The listing builds one solid part. Answer for the finished solid, in the listing's coordinates (mm). Face numbers are marked on the shaded views. A direction names the side the tool comes from. Coordinates: 2 decimals unless noted, no trailing zeros. Write each loop counter-clockwise with the first axis right and the second up, starting at its lowest first coordinate (ties: lowest second). Pieces come first, ordered by that corner, then holes.
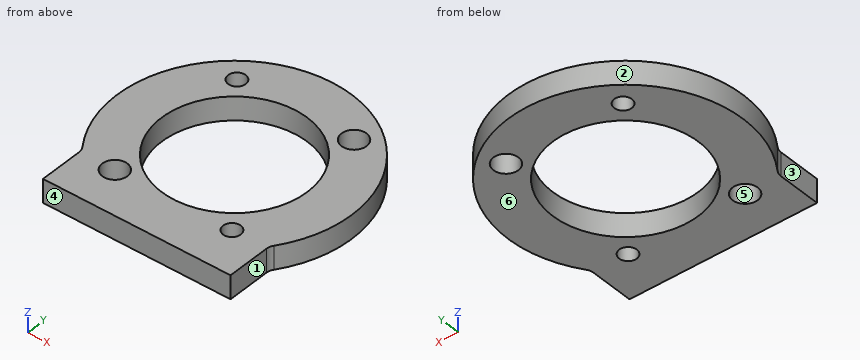
from build123d import *

# Parameters (mm, degrees)
SKETCH1_R           = 19.685
SKETCH1_R_2         = 2.38125
SKETCH1_R_3         = 3.3782
BOSS_EXTRUDE1_DEPTH = 6.35


with BuildPart() as part:
    # Sketch1 → Boss-Extrude1 (new body)
    with BuildSketch(Plane.XY):
        with BuildLine():
            Line((0, 0), (-50.8, 0))
            Line((-50.8, 0), (-50.8, 11.669536858))
            ThreePointArc((-50.8, 11.669536858), (-50.947756279, 12.626835377), (-51.377272727, 13.495033507))
            ThreePointArc((-51.377272727, 13.495033507), (-25.4, 63.5), (0.577272727, 13.495033507))
            ThreePointArc((0.577272727, 13.495033507), (0.147756279, 12.626835377), (0, 11.669536858))
            Line((0, 11.669536858), (0, 0))
        make_face()
        with Locations((-25.4, 31.75)):
            Circle(SKETCH1_R, mode=Mode.SUBTRACT)
        with Locations((-41.267254208, 51.58406776)):
            Circle(SKETCH1_R_2, mode=Mode.SUBTRACT)
        with Locations((-9.532745792, 51.58406776)):
            Circle(SKETCH1_R_3, mode=Mode.SUBTRACT)
        with Locations((-9.532745792, 11.91593224)):
            Circle(SKETCH1_R_2, mode=Mode.SUBTRACT)
        with Locations((-41.267254208, 11.91593224)):
            Circle(SKETCH1_R_3, mode=Mode.SUBTRACT)
    extrude(amount=BOSS_EXTRUDE1_DEPTH)


solid = part.part
Q1. Determine the mould class of the marked faces 4, 5 and 6 for opening direction Y: released by +Y, released by -Y, zero draft, split by the parting line, or undercut.
Answers below:
face 4: released by -Y
face 5: undercut
face 6: zero draft
Q2. The part is cut by section A-A, the plane x = -25.4. Write down the section's boundary in (y, z) (3 decimals).
Answers below:
outline: (0, 0) - (12.065, 0) - (12.065, 6.35) - (0, 6.35) - close; (51.435, 0) - (63.5, 0) - (63.5, 6.35) - (51.435, 6.35) - close
Q3. Find the intervals of material crossed by probe 1 along Y at (x, z) = (-43, 4.75); probe 2 along X at (y, z) = (52, 5); probe 3 along X at (y, z) = (10, 2), in increasing order.
Answers below:
probe 1: y = 0 to 9.02, 14.82 to 22.93, 40.57 to 49.95, 53.22 to 58.18
probe 2: x = -49.85 to -43.61, -38.92 to -12.89, -6.18 to -0.95
probe 3: x = -50.8 to -44.05, -38.48 to -10.95, -8.12 to 0
Q4. The part is cut by section C-C, the plane z = 4.5. State how many separate pieces and enclosed holes the cut face has, then the cut area to 3 significant figures.
Answers below:
separate pieces: 1
enclosed holes: 5
area: 2,040 mm2
Q5. Given pin 1 (11 mm diameter, centred on x = -9.53, y = 51.58, fed in from -Z); pin 2 (1.5 mm diameter, centred on y = 53, z = 5, fed in from -X); pin 3 (4.5 mm diameter, centred on x = -41.27, y = 51.58, fed in from -Z); pin 4 (1 mm diameter, centred on y = 21.5, z = 1.5, fed in from -X), each flat-ended and moving along its own axis, determine where each tip first touches the part or whether it passes through.
Answers below:
pin 1: stops at z = 0
pin 2: stops at x = -49.64
pin 3: passes through
pin 4: stops at x = -55.62
Q6. Which of the six approach directions +Z, -Z, +X, -X, +Y, -Y give full straight-line access (tool end or side, diameter ignored) to the marked faces 1, 2 and 3?
Answers below:
face 1: +Z, -Z, +X, -Y
face 2: +Z, -Z
face 3: +Z, -Z, -X, -Y
Q7. The part is cut by section D-D, the plane x = -2. Write down the section's boundary in (y, z), then the cut area to 3 significant figures.
Answers below:
outline: (0, 0) - (53.21, 0) - (53.21, 6.35) - (0, 6.35) - close
area: 338 mm2
Q8. The part is cut by section B-B, the plane y = 31.75. Write down the section's boundary in (x, z) (3 decimals), then the cut area to 3 significant figures.
Answers below:
outline: (-57.15, 0) - (-45.085, 0) - (-45.085, 6.35) - (-57.15, 6.35) - close; (-5.715, 0) - (6.35, 0) - (6.35, 6.35) - (-5.715, 6.35) - close
area: 153 mm2
